from build123d import *

# Parameters (mm, degrees)
SKETCH1_W           = 85
SKETCH1_H           = 14
BOSS_EXTRUDE1_DEPTH = 2
SKETCH2_W           = 85
SKETCH2_H           = 2
BOSS_EXTRUDE2_DEPTH = 6
SKETCH3_W           = 10
SKETCH3_H           = 10
BOSS_EXTRUDE3_DEPTH = 2
CUT_EXTRUDE1_DEPTH  = 4
CUT_EXTRUDE2_DEPTH  = 20
CHAMFER1_SIZE       = 1.5
SKETCH6_W           = 10
SKETCH6_H           = 10
BOSS_EXTRUDE4_DEPTH = 50
CUT_EXTRUDE3_DEPTH  = 50
FILLET1_R           = 10
CUT_EXTRUDE4_DEPTH  = 10


with BuildPart() as part:
    # Sketch1 → Boss-Extrude1 (new body)
    with BuildSketch(Plane.XY):
        with Locations((-9.558823529, 4.906862745)):
            Rectangle(SKETCH1_W, SKETCH1_H)
    extrude(amount=BOSS_EXTRUDE1_DEPTH)

    # Sketch2 → Boss-Extrude2 (add)
    with BuildSketch(Plane.XY):
        with Locations((-9.558823529, 10.906862745)):
            Rectangle(SKETCH2_W, SKETCH2_H)
    extrude(amount=BOSS_EXTRUDE2_DEPTH)

    # Sketch3 → Boss-Extrude3 (add)
    with BuildSketch(Plane(origin=(0, 0, 0), x_dir=(-1, 0, 0), z_dir=(0, 0, -1))):
        with Locations((-37.941176471, 2.906862745)):
            Rectangle(SKETCH3_W, SKETCH3_H)
    extrude(amount=-BOSS_EXTRUDE3_DEPTH)

    # Sketch4 → Cut-Extrude1 (cut)
    with BuildSketch(Plane.XY.offset(6)):
        Polygon((7.941176471, 9.906862745), (12.941176471, 11.906862745), (32.941176471, 11.906862745), (32.941176471, 9.906862745), align=None)
    extrude(amount=-CUT_EXTRUDE1_DEPTH, mode=Mode.SUBTRACT)

    # Sketch5 → Cut-Extrude2 (cut)
    with BuildSketch(Plane(origin=(0, 11.906862745, 0), x_dir=(1, 0, 0), z_dir=(0, 1, 0))):
        Polygon((-52.058823529, 0), (-36.428289141, -6), (-52.058823529, -6), align=None)
    extrude(amount=-CUT_EXTRUDE2_DEPTH, mode=Mode.SUBTRACT)

    # Chamfer1
    chamfer1_edges = [part.edges().sort_by_distance(p)[0] for p in [
        (-44.243556335, 11.906862745, 3),
    ]]
    chamfer(chamfer1_edges, length=CHAMFER1_SIZE)

    # Sketch6 → Boss-Extrude4 (add)
    with BuildSketch(Plane(origin=(42.941176471, 0, 0), x_dir=(0, 0, -1), z_dir=(1, 0, 0))):
        with Locations((-7, 2.906862745)):
            Rectangle(SKETCH6_W, SKETCH6_H)
    extrude(amount=-BOSS_EXTRUDE4_DEPTH)

    # Sketch7 → Cut-Extrude3 (cut)
    with BuildSketch(Plane.XZ.offset(2.093137255)):
        Polygon((42.941176471, 0), (38.092861761, 12), (42.941176471, 12), align=None)
    extrude(amount=-CUT_EXTRUDE3_DEPTH, mode=Mode.SUBTRACT)

    # Fillet1
    fillet1_edges = [part.edges().sort_by_distance(p)[0] for p in [
        (40.517019116, -2.093137255, 6),
    ]]
    fillet(fillet1_edges, radius=FILLET1_R - 0.0001)  # a hair under: the kernel refuses the full size

    # Sketch8 → Cut-Extrude4 (cut)
    with BuildSketch(Plane.XY.offset(12)):
        with BuildLine():
            Line((-7.058823529, -2.093137255), (-7.058823529, 7.906862745))
            Line((-7.058823529, 7.906862745), (38.092861761, 7.906862745))
            add(Edge.make_bspline(
                [(-7.058823529, -2.093137255), (8.253894017, -0.195900436), (26.879326583, -4.673987429), (38.092861761, 7.906862745)],
                knots=[0, 0, 0, 0, 1, 1, 1, 1], degree=3))
        make_face()
    extrude(amount=-CUT_EXTRUDE4_DEPTH, mode=Mode.SUBTRACT)


solid = part.part
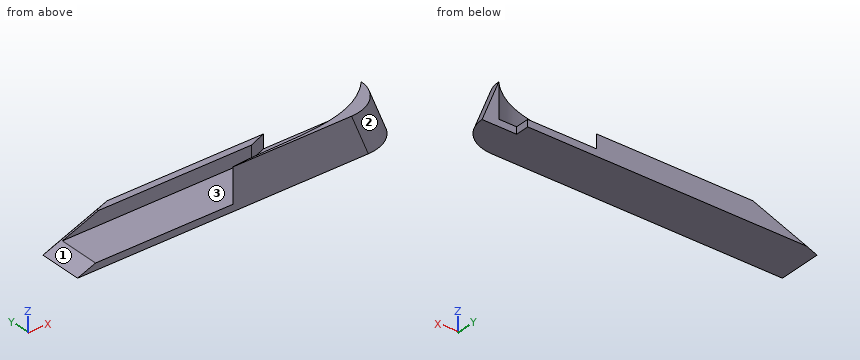
Geometry: final body of the model. Coordinates: model frame, mm. Face numbers are marked on the shaded views. Coordinates: 2 decimals unless noted, no trailing zeros. Order: outer loops, then holes, each group sorted by start corner. A loop starts at its lowest first (then second) coordinate and runs counter-clockwise, first axis right, second up.
1) Section A-A (x = -14). Return loops of the section in (y, z).
Result sheet:
outline: (-2.09, 0) - (11.91, 0) - (11.91, 6) - (9.91, 6) - (9.91, 2) - (-2.09, 2) - close
2) Section D-D (x = -45). Return loops of the section in (y, z).
Result sheet:
outline: (-2.09, 0) - (11.91, 0) - (11.91, 1.1) - (10.41, 2.71) - (9.91, 2.71) - (9.91, 2) - (-2.09, 2) - close
3) Ray query, probe 1 along Z at (x, y) = (-17, 10.75); probe 2 along Y at (x, z) = (-41, 2.25); probe 3 along Z at (x, y) = (-1, 2.25). Return the intervals inside material, ascending.
Result sheet:
probe 1: z = 0 to 6
probe 2: y = 9.91 to 11.91
probe 3: z = 0 to 2
4) Draft query along Y for the marked faces 1, 2 and 3. Return one class per face: released by +Y, released by -Y, zero draft, split by the parting line, or undercut.
Result sheet:
face 1: zero draft
face 2: released by -Y
face 3: undercut
5) Section B-B (y = 8.75). Return loops of the section in (x, z), then the cut area to 3 significant figures.
Result sheet:
outline: (-52.06, 0) - (32.94, 0) - (32.94, 2) - (-46.85, 2) - close
area: 165 mm2
6) First-contact query: P1, Ø1, axis at y = 10, z = 1.5, coming from the +X side; P2, Ø3, axis at y = 8.5, z = 4, coming from the +X side; P3, Ø3, axis at x = 39, z = 8, coming from the +Y side. Flat tips, straight axial feed; report the tip coordinate or a pass-through.
Result sheet:
P1: stops at x = 32.94
P2: stops at x = 41.88
P3: stops at y = 7.91
7) Section C-C (x = -34.5). Return loops of the section in (y, z), then the cut area to 3 significant figures.
Result sheet:
outline: (-2.09, 0) - (11.91, 0) - (11.91, 5.13) - (11.1, 6) - (9.91, 6) - (9.91, 2) - (-2.09, 2) - close
area: 35.6 mm2
